For this review, take the finished solid that the model builds, in its own axes (mm). Round coordinates to 2 decimals unless told otherwise and drop trailing zeros. Order: outer loops, then holes, each group sorted by start corner. A loop starts at its lowest first (then second) coordinate and runs counter-clockwise, first axis right, second up. Notation, with made-up numbers: (-2, 74) -> (19, 74) arc R20 cw to (19, 100) -> close; hole circle Ø4 at (49, 41). An arc over 180 degrees is marked (long way). Answer in a Markdown table with one row per item.
```python
from build123d import *

# Parameters (mm, degrees)
SKETCH1_W                    = 82.55
SKETCH1_H                    = 50.8
BOSS_EXTRUDE1_DEPTH          = 12.7
F_10_0_1935_DIAMETER_HOLE1_D = 4.9149
F_4_40_TAPPED_HOLE1_D        = 2.2606


with BuildPart() as part:
    # Sketch1 → Boss-Extrude1 (new, symmetric)
    with BuildSketch(Plane(origin=(0, 0, 0), x_dir=(0, 0, -1), z_dir=(1, 0, 0))):
        Rectangle(SKETCH1_W, SKETCH1_H)
    extrude(amount=BOSS_EXTRUDE1_DEPTH, both=True)

    # #10 (0.1935) Diameter Hole1 (through all)
    with Locations(Plane(origin=(12.7, 0, 0), x_dir=(0, 0, -1), z_dir=(1, 0, 0))):
        with Locations((28.575, 12.7), (-28.575, 12.7), (-28.575, -12.7), (28.575, -12.7)):
            Hole(F_10_0_1935_DIAMETER_HOLE1_D / 2)

    # #4-40 Tapped Hole1 (through all)
    with Locations(Plane(origin=(12.7, 0, 0), x_dir=(0, 0, -1), z_dir=(1, 0, 0))):
        with Locations((0, 19.05), (0, 12.7), (0, 6.35), (0, 0), (0, -6.35), (0, -12.7), (0, -19.05)):
            Hole(F_4_40_TAPPED_HOLE1_D / 2)


solid = part.part
```
Q1. Take a section at C-C, the plane y = -6.35. Write out the cut boundary in (x, z) (3 decimals).
Answer key:
| item | result |
|---|---|
| outline | (-12.7, -41.275) -> (12.7, -41.275) -> (12.7, -1.13) -> (-12.7, -1.13) -> close; (-12.7, 1.13) -> (12.7, 1.13) -> (12.7, 41.275) -> (-12.7, 41.275) -> close |
Q2. Take a section at A-A, the plane y = -12.7. Write out the cut boundary in (x, z) (3 decimals), then the cut area to 3 significant figures.
Answer key:
| item | result |
|---|---|
| outline | (-12.7, -41.275) -> (12.7, -41.275) -> (12.7, -31.032) -> (-12.7, -31.032) -> close; (-12.7, -26.118) -> (12.7, -26.118) -> (12.7, -1.13) -> (-12.7, -1.13) -> close; (-12.7, 1.13) -> (12.7, 1.13) -> (12.7, 26.118) -> (-12.7, 26.118) -> close; (-12.7, 31.032) -> (12.7, 31.032) -> (12.7, 41.275) -> (-12.7, 41.275) -> close |
| area | 1,790 mm^2 |
Q3. To check wall thickness, follow probe 1 along Y at (x, z) = (-10.75, 30); probe 2 along Y at (x, z) = (3.5, 26.5). State the ranges of each line that lie inside material, in increasing order.
Answer key:
| item | result |
|---|---|
| probe 1 | y = -25.4 to -14.7, -10.7 to 10.7, 14.7 to 25.4 |
| probe 2 | y = -25.4 to -14.02, -11.38 to 11.38, 14.02 to 25.4 |
Q4. Take a section at D-D, the plane z = -27. Write out the cut boundary in (x, y).
Answer key:
| item | result |
|---|---|
| outline | (-12.7, -25.4) -> (12.7, -25.4) -> (12.7, -14.59) -> (-12.7, -14.59) -> close; (-12.7, -10.81) -> (12.7, -10.81) -> (12.7, 10.81) -> (-12.7, 10.81) -> close; (-12.7, 14.59) -> (12.7, 14.59) -> (12.7, 25.4) -> (-12.7, 25.4) -> close |
Q5. Clearance check with a flat-ended pin moving along its axis: pin 1 Ø8 at (y, z) = (12.7, -28.575) entering from +X. State where the tip first meets the part, or that it passes through.
Answer key:
| item | result |
|---|---|
| pin 1 | stops at x = 12.7 |
Q6. Take a section at B-B, the plane x = -0.25. Give the number of separate pieces and of enclosed holes in the cut face, then the cut area to 3 significant figures.
Answer key:
| item | result |
|---|---|
| separate pieces | 1 |
| enclosed holes | 11 |
| area | 4,090 mm^2 |
Q7. The part is to be moulded in two halves that separate along Y. For faces 1 (the face through (0, 0, 41.275)), 2 (the face through (-0.178, -1.103, -0.245)), 3 (the face through (0, 25.4, 1)), say which applies: +Y half, -Y half, draft (parallel to the pull), parting line (faces both ways), or undercut.
Answer key:
| item | result |
|---|---|
| face 1 | draft |
| face 2 | undercut |
| face 3 | +Y half |
